For this review, use the dimensioned drawing (mm, ordinates from the lowest corner) and the shaded views. Coordinates: 2 decimals unless noted, no trailing zeros. Write each loop counter-clockwise with the first axis right and the second up, starting at its lowest first coordinate (ties: lowest second). Pieces come first, ordered by that corner, then holes.
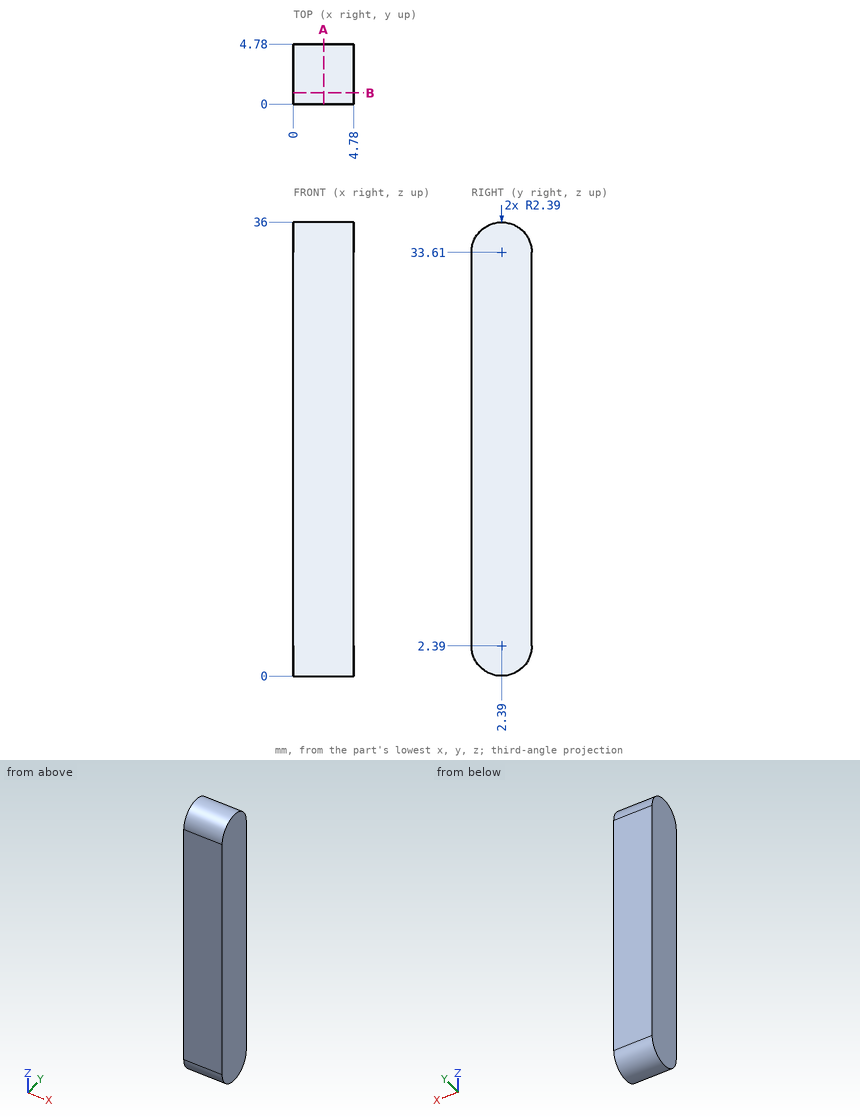
Item 1: For pin 1 (1.5 mm diameter, centred on x = 2.5, y = 3.5, fed in from -Z), flat-tipped, find the tip position at first contact; note if it passes through.
Solved:
pin 1: stops at z = 0.03
Item 2: Take a section at A-A, the plane x = 2.4. Write out the cut boundary in (y, z), plus the area to 3 significant figures.
Solved:
outline: (0, 2.39) arc R2.39 ccw to (4.78, 2.39) - (4.78, 33.61) arc R2.39 ccw to (0, 33.61) - close
area: 167 mm2
Item 3: Take a section at B-B, the plane y = 0.9. Write out the cut boundary in (x, z).
Solved:
outline: (0, 0.52) - (4.78, 0.52) - (4.78, 35.48) - (0, 35.48) - close
Item 4: To check wall thickness, follow line 1 along Z through (x, y) = (4.1, 2.2); line 2 along Z through (x, y) = (0.95, 0.95). State the ranges of each line that lie inside material, in increasing order.
Solved:
line 1: z = 0.01 to 35.99
line 2: z = 0.48 to 35.52
